Autodesk Inventor part; units mm, degrees
ref_plane "YZ Plane" through (0, 0, 0) normal (1, 0, 0) x (0, 1, 0)
ref_plane "XZ Plane" through (0, 0, 0) normal (0, 1, 0) x (-1, 0, 0)
ref_plane "XY Plane" through (0, 0, 0) normal (0, 0, 1) x (1, 0, 0)
sketch "Sketch1" plane through (0, 0, 0) normal (0, 0, 1) x (1, 0, 0)
  line L0 (0, 0) -> (12.7, 0)
  line L1 (12.7, 0) -> (12.7, 31.75)
  line L2 (12.7, 31.75) -> (0, 31.75)
  line L3 (0, 12.7) -> (0, 0)
  line L4 (12.7, 31.75) -> (-12.7, 31.75)
  line L5 (-12.7, 31.75) -> (-12.7, 12.7)
  line L6 (-12.7, 12.7) -> (0, 12.7)
  line L7 (12.7, 12.7) -> (12.7, 31.75)
  dimension "d1" = 31.75
  dimension "d2" = 25.4
  dimension "d3" = 19.05
  dimension "d4" = 12.7
  dimension "d5" = 12.7
extrude "Extrusion1" add sketch "Sketch1" along normal blind 6.35
fillet "Fillet1" radius 19.05 1 edges at (-12.7, 31.75, 3.175)
sketch "Sketch2" plane through (0, 0, 6.35) normal (0, 0, 1) x (1, 0, 0)
  line L0 (12.7, 0) -> (12.7, 31.75)
  line L1 (0, 0) -> (12.7, 0)
  point P0 (6.35, 6.35)
  dimension "d11" = 6.35
  dimension "d12" = 6.35
hole "Hole1" at (6.35, 6.35, 6.35) direction (0, 0, -1) diameter 6.604 end through all
sketch "Sketch3" plane through (0, 0, 6.35) normal (0, 0, 1) x (1, 0, 0)
  line L0 (12.7, 0) -> (12.7, 31.75)
  line L1 (12.7, 31.75) -> (6.35, 31.75)
  point P0 (0, 0)
  point P1 (6.35, 25.4)
  dimension "d20" = 6.35
  dimension "d21" = 6.35
hole "Hole2" at (6.35, 25.4, 6.35) direction (0, 0, -1) diameter 3.556 end through all
sketch "Sketch4" plane through (0, 0, 6.35) normal (0, 0, 1) x (1, 0, 0)
  circle A0 centre (6.35, 6.35) radius 3.302
  circle A1 centre (6.35, 6.35) radius 19.05
  line L0 (-7.1204, 19.8204) -> (6.35, 6.35)
  line L1 (12.7, 0) -> (12.7, 31.75)
  point P0 (0, 0)
  dimension "d29" = 38.1
  dimension "d30" = 45
hole "Hole3" at (-7.1204, 19.8204, 6.35) direction (0, 0, -1) diameter 3.81 end through all
properties part number "Shooter_Stop"
Check sheet for the modelled part. Datum: model origin and axes. Units: mm. A direction names the side the tool comes from. Round coordinates to 2 decimals unless told otherwise and drop trailing zeros. Write each loop counter-clockwise with the first axis right and the second up, starting at its lowest first coordinate (ties: lowest second). Pieces come first, ordered by that corner, then holes. Notation, with made-up numbers: (14, 13) -> (50, 13) arc R21 ccw to (50, 18) -> close; hole circle Ø8 at (50.5, 33). An arc over 180 degrees is marked (long way). Answer as CSV lines item,"result". Start each with the question number.
1) Release check for a two-part mould opening along Y. For faces 1 (the cylindrical face through (8.086, 25.785, 3.131)), 2 (the flat face through (6, 0, 3)), 3 (the flat face through (3, 20, 0)) record: pulls with the +Y half, pulls with the -Y half, needs draft (parallel to the pull), parting line crosses it, or undercut.
2) Section check D-D on y = 10.5. Enter the section's corners in (x, z), and give its area (3 significant figures).
3) Tool access check on faces 4 (the flat face through (3, 20, 6.35)), 5 (the flat face through (0, 6, 3)). Record the directions out of +Z, -Z, +X, -X, +Y, -Y that give a thin tool (end or side, any length) a straight path to the whole face; none if there is none.
4) Section check A-A on y = 6.35. Enter the section's corners in (x, z).
5) Section check C-C on z = 4. State how many separate pieces and enclosed holes the cut face has, and give its area (3 significant figures).
6) Material ranges on line 1 (Y direction, x = 6.35, z = 3.25); line 2 (Y direction, x = 6.5, z = 4.75); line 3 (X direction, y = 6.35, z = 2.5), recorded low to high. Write a range as from..to.
7) Section check B-B on x = 7.25. Enter the section's corners in (y, z), and give its area (3 significant figures).
Found:
1,face 1,"undercut"
1,face 2,"pulls with the -Y half"
1,face 3,"needs draft"
2,outline,"(0, 0) -> (12.7, 0) -> (12.7, 6.35) -> (0, 6.35) -> close"
2,area,"80.6 mm^2"
3,face 4,"+Z, +X, -X, +Y, -Y"
3,face 5,"+Z, -Z, -X, -Y"
4,outline,"(0, 0) -> (3.05, 0) -> (3.05, 6.35) -> (0, 6.35) -> close; (9.65, 0) -> (12.7, 0) -> (12.7, 6.35) -> (9.65, 6.35) -> close"
5,separate pieces,"1"
5,enclosed holes,"3"
5,area,"512 mm^2"
6,line 1,"y = 0..3.05, 9.65..23.62, 27.18..31.75"
6,line 2,"y = 0..3.05, 9.65..23.63, 27.17..31.75"
6,line 3,"x = 0..3.05, 9.65..12.7"
7,outline,"(0, 0) -> (3.17, 0) -> (3.17, 6.35) -> (0, 6.35) -> close; (9.53, 0) -> (23.87, 0) -> (23.87, 6.35) -> (9.53, 6.35) -> close; (26.93, 0) -> (31.75, 0) -> (31.75, 6.35) -> (26.93, 6.35) -> close"
7,area,"142 mm^2"
